CAD build for the part. Positions are in the model's coordinates, mm. Give positions to 0.01 mm unless a question says otherwise; leave off trailing zeros. Order: outer loops, then holes, each group sorted by start corner. A loop starts at its lowest first (then second) coordinate and runs counter-clockwise, first axis right, second up.
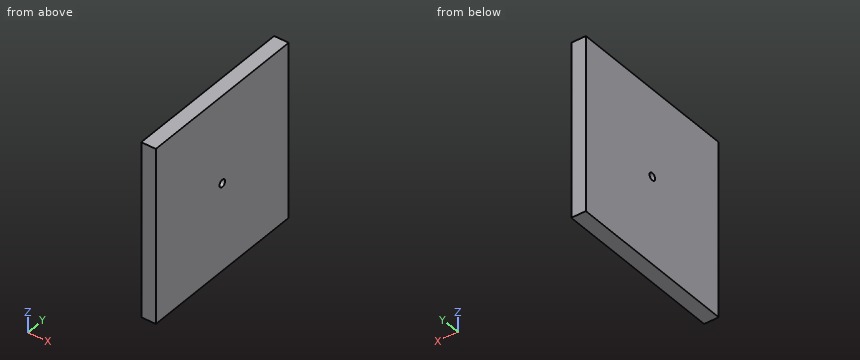
from build123d import *

# Parameters (mm, degrees)
SKETCH1_W               = 304.8
SKETCH1_H               = 304.8
BOSS_EXTRUDE1_DEPTH     = 12.7
SKETCH2_R               = 6.35
CUT_EXTRUDE1_DEPTH      = 13.7
CUT_EXTRUDE1_DEPTH_BACK = 13.7


with BuildPart() as part:
    # Sketch1 → Boss-Extrude1 (new body, symmetric)
    with BuildSketch(Plane(origin=(0, 0, 0), x_dir=(0, 0, -1), z_dir=(1, 0, 0))):
        Rectangle(SKETCH1_W, SKETCH1_H)
    extrude(amount=BOSS_EXTRUDE1_DEPTH, both=True)

    # Sketch2 → Cut-Extrude1 (cut, two sides)
    with BuildSketch(Plane(origin=(0, 0, 0), x_dir=(0, 0, -1), z_dir=(1, 0, 0))) as cut_extrude1_sk:
        Circle(SKETCH2_R)
    extrude(amount=CUT_EXTRUDE1_DEPTH, mode=Mode.SUBTRACT)
    extrude(cut_extrude1_sk.sketch, amount=-CUT_EXTRUDE1_DEPTH_BACK, mode=Mode.SUBTRACT)


solid = part.part
1. Wall check: line 1 (Y direction, x = 4.25, z = 0); line 2 (Z direction, x = -0.25, y = 5). Give the ranges that are in metal, low to high.
2. Saw through at A-A on y = 0. Give the cut face in (x, z).
Reported:
1. line 1: y = -152.4 to -6.35, 6.35 to 152.4
1. line 2: z = -152.4 to -3.91, 3.91 to 152.4
2. outline: (-12.7, -152.4) - (12.7, -152.4) - (12.7, -6.35) - (-12.7, -6.35) - close; (-12.7, 6.35) - (12.7, 6.35) - (12.7, 152.4) - (-12.7, 152.4) - close
